from build123d import *

# Parameters (mm, degrees)
SKETCH1_W             = 42
SKETCH1_H             = 42
SKETCH1_R             = 3.407851421
BOSS_EXTRUDE1_DEPTH   = 46.75
SKETCH2_R             = 10.95
BOSS_EXTRUDE2_DEPTH   = 2
CUT_EXTRUDE1_START    = -8
CUT_EXTRUDE1_DEPTH    = 30
CIRPATTERN1_COUNT     = 4
FILLET1_R             = 3
CHAMFER1_SIZE         = 4
FILLET2_R             = 3
SKETCH4_R             = 4.65
CUT_EXTRUDE2_DEPTH    = 2.4
DELETEFACE1_OUTLINE_R = 3.407851421
DELETEFACE1_DEPTH     = 46.35
SKETCH5_R             = 2.5
BOSS_EXTRUDE3_DEPTH   = 23.25
CUT_EXTRUDE3_DEPTH    = 15.25
SKETCH7_R             = 0.875
CUT_EXTRUDE4_DEPTH    = 2
SKETCH8_R             = 1.5
CUT_EXTRUDE5_DEPTH    = 5


# Read off the part's stored shape, not the designer's step: DeleteFace1
with BuildPart() as part:
    # Sketch1 → Boss-Extrude1 (new body)
    with BuildSketch(Plane(origin=(0, 0, 0), x_dir=(1, 0, 0), z_dir=(0, 1, 0))):
        Rectangle(SKETCH1_W, SKETCH1_H)
        with Locations(Location((0, 0, 0), (0, 0, 270))):
            Circle(SKETCH1_R, mode=Mode.SUBTRACT)
    extrude(amount=BOSS_EXTRUDE1_DEPTH)

    # Sketch2 → Boss-Extrude2 (add)
    with BuildSketch(Plane(origin=(0, 46.75, 0), x_dir=(1, 0, 0), z_dir=(0, 1, 0))):
        with Locations(Location((0, 0, 0), (0, 0, 90))):
            Circle(SKETCH2_R)
    extrude(amount=BOSS_EXTRUDE2_DEPTH)

    # Sketch3 → Cut-Extrude1 (cut)
    with BuildSketch(Plane(origin=(0, 46.75, 0), x_dir=(1, 0, 0), z_dir=(0, 1, 0)).offset(CUT_EXTRUDE1_START)):
        with BuildLine():
            Line((-14.355339059, 21), (-21, 21))
            Line((-21, 21), (-21, 14.355339059))
            ThreePointArc((-21, 14.355339059), (-17.901682199, 17.901682199), (-14.355339059, 21))
        make_face()
    cut_extrude1 = extrude(amount=-CUT_EXTRUDE1_DEPTH, mode=Mode.SUBTRACT)

    # CirPattern1: Cut-Extrude1 ×4 about axis
    cirpattern1_axis = Axis((0, 0, 0), (0, 1, 0))
    for i in range(1, CIRPATTERN1_COUNT):
        add(cut_extrude1.rotate(cirpattern1_axis, i * 360 / CIRPATTERN1_COUNT), mode=Mode.SUBTRACT)

    # Fillet1
    fillet1_edges = [part.edges().sort_by_distance(p)[0] for p in [
        (-14.355339059, 23.75, -21),
        (-21, 23.75, -14.355339059),
        (21, 23.75, -14.355339059),
        (14.355339059, 23.75, -21),
        (14.355339059, 23.75, 21),
        (21, 23.75, 14.355339059),
        (-21, 23.75, 14.355339059),
        (-14.355339059, 23.75, 21),
    ]]
    fillet(fillet1_edges, radius=FILLET1_R)

    # Chamfer1
    chamfer1_edges = [part.edges().sort_by_distance(p)[0] for p in [
        (-21, 4.375, -21),
        (21, 4.375, -21),
        (21, 4.375, 21),
        (-21, 4.375, 21),
        (-21, 42.75, -21),
        (-21, 42.75, 21),
        (21, 42.75, 21),
        (21, 42.75, -21),
    ]]
    chamfer(chamfer1_edges, length=CHAMFER1_SIZE)

    # Fillet2
    fillet2_edges = [part.edges().sort_by_distance(p)[0] for p in [
        (17, 42.75, 21),
        (17, 4.375, 21),
        (-17, 4.375, 21),
        (-17, 42.75, 21),
        (-21, 42.75, -17),
        (-21, 4.375, -17),
        (-21, 4.375, 17),
        (-21, 42.75, 17),
        (17, 42.75, -21),
        (17, 4.375, -21),
        (-17, 42.75, -21),
        (-17, 4.375, -21),
        (21, 42.75, -17),
        (21, 4.375, -17),
        (21, 42.75, 17),
        (21, 4.375, 17),
    ]]
    fillet(fillet2_edges, radius=FILLET2_R)

    # Sketch4 → Cut-Extrude2 (cut)
    with BuildSketch(Plane(origin=(0, 48.75, 0), x_dir=(1, 0, 0), z_dir=(0, 1, 0))):
        with Locations(Location((0, 0, 0), (0, 0, 270))):
            Circle(SKETCH4_R)
    extrude(amount=-CUT_EXTRUDE2_DEPTH, mode=Mode.SUBTRACT)

    # DeleteFace1 outline → DeleteFace1 (add)
    with BuildSketch(Plane(origin=(0, 0, 0), x_dir=(1, 0, 0), z_dir=(0, 1, 0))):
        Circle(DELETEFACE1_OUTLINE_R)
    extrude(amount=DELETEFACE1_DEPTH)

    # Sketch5 → Boss-Extrude3 (add)
    with BuildSketch(Plane(origin=(0, 46.35, 0), x_dir=(1, 0, 0), z_dir=(0, 1, 0))):
        with Locations(Location((0, 0, 0), (0, 0, 90))):
            Circle(SKETCH5_R)
    extrude(amount=BOSS_EXTRUDE3_DEPTH)

    # Sketch6 → Cut-Extrude3 (cut)
    with BuildSketch(Plane(origin=(0, 69.6, 0), x_dir=(1, 0, 0), z_dir=(0, 1, 0))):
        with BuildLine():
            Line((-2, 1.5), (-2, -1.5))
            ThreePointArc((-2, -1.5), (-10.750577437, 0), (-2, 1.5))
        make_face()
    extrude(amount=-CUT_EXTRUDE3_DEPTH, mode=Mode.SUBTRACT)

    # Sketch7 → Cut-Extrude4 (cut)
    with BuildSketch(Plane(origin=(0, 69.6, 0), x_dir=(1, 0, 0), z_dir=(0, 1, 0))):
        with Locations(Location((0, 0, 0), (0, 0, 270))):
            Circle(SKETCH7_R)
    extrude(amount=-CUT_EXTRUDE4_DEPTH, mode=Mode.SUBTRACT)

    # Sketch8 → Cut-Extrude5 (cut)
    with BuildSketch(Plane(origin=(0, 46.75, 0), x_dir=(1, 0, 0), z_dir=(0, 1, 0))):
        with Locations(Location((-15.556349186, 15.556349186, 0), (0, 0, 270))):
            Circle(SKETCH8_R)
        with Locations(Location((15.556349186, 15.556349186, 0), (0, 0, 270))):
            Circle(SKETCH8_R)
        with Locations(Location((15.556349186, -15.556349186, 0), (0, 0, 270))):
            Circle(SKETCH8_R)
        with Locations(Location((-15.556349186, -15.556349186, 0), (0, 0, 270))):
            Circle(SKETCH8_R)
    extrude(amount=-CUT_EXTRUDE5_DEPTH, mode=Mode.SUBTRACT)


solid = part.part
Build history of the part. All positions in model axes, mm. A direction names the side the tool comes from. Round coordinates to 2 decimals unless told otherwise and drop trailing zeros. Loops run counter-clockwise (first coordinate to the right, second up) from the corner with the lowest first, then second, coordinate; pieces in that order, holes last. Notation, with made-up numbers: (35, -17) -> (89, -17) arc R13 cw to (89, -6) -> close; hole circle Ø9 at (18, 8). An arc over 180 degrees is marked (long way). One line per item, written item: value. Start each with the question number.
Q1. Two-plate mould, pull along X, no slides. Class faces 1 (the face through (20.765, 42.806, 16.921)), 2 (the face through (-17.938, 23.96, -17.866)), 3 (the face through (-16, 41.75, -16)): released by +X, released by -X, zero draft, split by the parting line, or undercut.
Q2. Drop flat-ended pins along their axis: pin 1 Ø3.5 at (x, z) = (15.5, -16) entering from +Y; pin 2 Ø0.9 at (x, z) = (15, 16) entering from +Y; pin 3 Ø2 at (x, y) = (0.5, 62.5) entering from +Z. Give the stop position or say it passes through.
Q3. Cut at C-C on z = 0. List the corners of the cut face in (x, y) (3 decimals), plus the area to 3 significant figures.
Q4. Cut at A-A on y = 7.5. List the corners of the cut face in (x, z), plus the area to 3 significant figures.
Q5. Cut at B-B on x = 0. List the corners of the cut face in (y, z) (3 decimals), plus the area to 3 significant figures.
Q6. Cut at D-D on y = 27. List the corners of the cut face in (x, z), plus the area to 3 significant figures.
Q7. Probe line 1 along X through (y, z) = (47, 0); line 2 along X through (y, z) = (68.8, 0) (3 decimals); line 3 along Z through (x, y) = (2, 61.5). List the from-to ranges inside material, lowest first.
Q8. 3-axis set-ups, long thin cutter, end or side, ignore diameter. For faces 4 (the face through (-20.78, 4.44, -16.89)), 5 (the face through (-18.3, 8.75, -18)), 6 (the face through (20.83, 23.54, -14.31)), 7 (the face through (16, 41.75, -16)), 8 (the face through (-18, 38.75, 18.3)): which of +Z, -Z, +X, -X, +Y, -Y reach the whole face in a straight line?
Computed:
1. face 1: released by +X
1. face 2: released by -X
1. face 3: undercut
2. pin 1: y = 46.75
2. pin 2: y = 41.75
2. pin 3: z = 2.5
3. outline: (-21, 0) -> (21, 0) -> (21, 46.75) -> (10.95, 46.75) -> (10.95, 48.75) -> (4.65, 48.75) -> (4.65, 46.35) -> (2.5, 46.35) -> (2.5, 69.6) -> (0.875, 69.6) -> (0.875, 67.6) -> (-0.875, 67.6) -> (-0.875, 69.6) -> (-2, 69.6) -> (-2, 54.35) -> (-2.5, 54.35) -> (-2.5, 46.35) -> (-4.65, 46.35) -> (-4.65, 48.75) -> (-10.95, 48.75) -> (-10.95, 46.75) -> (-21, 46.75) -> close
3. area: 2,090 mm²
4. outline: (-21, -15.76) arc R3 ccw to (-20.12, -17.88) -> (-17.88, -20.12) arc R3 ccw to (-15.76, -21) -> (15.76, -21) arc R3 ccw to (17.88, -20.12) -> (20.12, -17.88) arc R3 ccw to (21, -15.76) -> (21, 15.76) arc R3 ccw to (20.12, 17.88) -> (17.88, 20.12) arc R3 ccw to (15.76, 21) -> (-15.76, 21) arc R3 ccw to (-17.88, 20.12) -> (-20.12, 17.88) arc R3 ccw to (-21, 15.76) -> close
4. area: 1,730 mm²
5. outline: (0, -21) -> (46.75, -21) -> (46.75, -10.95) -> (48.75, -10.95) -> (48.75, -4.65) -> (46.35, -4.65) -> (46.35, -2.5) -> (69.6, -2.5) -> (69.6, -0.875) -> (67.6, -0.875) -> (67.6, 0.875) -> (69.6, 0.875) -> (69.6, 2.5) -> (46.35, 2.5) -> (46.35, 4.65) -> (48.75, 4.65) -> (48.75, 10.95) -> (46.75, 10.95) -> (46.75, 21) -> (0, 21) -> close
5. area: 2,100 mm²
6. outline: (-21, -13.32) arc R3 ccw to (-20.33, -15.21) arc R35 ccw to (-15.21, -20.33) arc R3 ccw to (-13.32, -21) -> (13.32, -21) arc R3 ccw to (15.21, -20.33) arc R35 ccw to (20.33, -15.21) arc R3 ccw to (21, -13.32) -> (21, 13.32) arc R3 ccw to (20.33, 15.21) arc R35 ccw to (15.21, 20.33) arc R3 ccw to (13.32, 21) -> (-13.32, 21) arc R3 ccw to (-15.21, 20.33) arc R35 ccw to (-20.33, 15.21) arc R3 ccw to (-21, 13.32) -> close
6. area: 1,680 mm²
7. line 1: -10.95 to -4.65, -2.5 to 2.5, 4.65 to 10.95
7. line 2: -2 to -0.875, 0.875 to 2.5
7. line 3: -1.5 to 1.5
8. face 4: -Z, -X, +Y, -Y
8. face 5: -Z, -X
8. face 6: -Z, +X
8. face 7: +Y
8. face 8: +Z, -X
